Input: part model. Units: mm. Frame: model coordinates. A direction names the side the tool comes from. Coordinates: 2 decimals unless noted, no trailing zeros. Order: outer loops, then holes, each group sorted by start corner. A loop starts at its lowest first (then second) coordinate and runs counter-clockwise, first axis right, second up.
from build123d import *

# Parameters (mm, degrees)
SKETCH1_R               = 1.375
BOSS_EXTRUDE1_DEPTH     = 6.25
CUT_EXTRUDE1_DEPTH      = 15.811313244
CUT_EXTRUDE1_DEPTH_BACK = 15.811313244
SKETCH2_W               = 8
SKETCH2_H               = 6.5
BOSS_EXTRUDE2_START     = -10
BOSS_EXTRUDE2_OUTLINE_W = 11.434309127
BOSS_EXTRUDE2_OUTLINE_H = 8.5
BOSS_EXTRUDE2_DEPTH     = 20
FILLET4_R               = 1.5
FILLET5_R               = 1.5
FILLET6_R               = 3
CUT_EXTRUDE2_DEPTH      = 0.1


# Read off the part's stored shape, not the designer's step: Boss-Extrude2
with BuildPart() as part:
    # Sketch1 → Boss-Extrude1 (new, symmetric)
    with BuildSketch(Plane.XY):
        with BuildLine():
            Line((-10, 5.5), (-10, -3))
            Line((-10, -3), (8, -3))
            ThreePointArc((8, -3), (12.25, 1.25), (8, 5.5))
            Line((8, 5.5), (-10, 5.5))
        make_face()
        with Locations((8, 1.25)):
            Circle(SKETCH1_R, mode=Mode.SUBTRACT)
    extrude(amount=BOSS_EXTRUDE1_DEPTH, both=True)

    # Sketch2 → Cut-Extrude1 (cut, two sides: drawn at the far end of the back side and taken through both)
    with BuildSketch(Plane(origin=(0, 0, 0), x_dir=(1, 0, 0), z_dir=(0, 1, 0)).offset(-CUT_EXTRUDE1_DEPTH_BACK)):
        with Locations((8.25, 1)):
            Rectangle(SKETCH2_W, SKETCH2_H)
    extrude(amount=CUT_EXTRUDE1_DEPTH + CUT_EXTRUDE1_DEPTH_BACK, mode=Mode.SUBTRACT)

    # Boss-Extrude2 outline → Boss-Extrude2 (add)
    with BuildSketch(Plane.XY.offset(BOSS_EXTRUDE2_START)):
        with Locations((-4.282845436, 1.25)):
            Rectangle(BOSS_EXTRUDE2_OUTLINE_W, BOSS_EXTRUDE2_OUTLINE_H)
    extrude(amount=BOSS_EXTRUDE2_DEPTH)

    # Sketch1<5> → Cut-Revolve2 (revolve, cut)
    with BuildSketch(Plane.XY):
        with BuildLine():
            Line((-9.391951793, 2.5), (-10, 2.5))
            Line((-10, 2.5), (-10, 0))
            Line((-10, 0), (-7.720367157, 0))
            ThreePointArc((-7.720367157, 0), (-7.220367157, 0.5), (-6.720367157, 0))
            Line((-6.720367157, 0), (-2.720367157, 0))
            ThreePointArc((-2.720367157, 0), (-2.220367157, 0.5), (-1.720367157, 0))
            Line((-1.720367157, 0), (0, 0))
            Line((0, 0), (0, 2.5))
            Line((0, 2.5), (-3.391951793, 2.5))
            ThreePointArc((-3.391951793, 2.5), (-3.891951793, 2), (-4.391951793, 2.5))
            Line((-4.391951793, 2.5), (-8.391951793, 2.5))
            ThreePointArc((-8.391951793, 2.5), (-8.891951793, 2), (-9.391951793, 2.5))
        make_face()
    revolve(axis=Axis((-50, 0, 0), (0, 1, 0)), mode=Mode.SUBTRACT)

    # Fillet4
    fillet4_edges = [part.edges().sort_by_distance(p)[0] for p in [
        (4.25, 1.25, 2.25),
        (4.25, 1.25, -4.25),
    ]]
    fillet(fillet4_edges, radius=FILLET4_R)

    # Fillet5
    fillet5_edges = [part.edges().sort_by_distance(p)[0] for p in [
        (1.434309127, 1.25, -6.25),
        (1.434309127, 1.25, 6.25),
        (-1.010205144, 1.25, 10),
        (-1.010205144, 1.25, -10),
    ]]
    fillet(fillet5_edges, radius=FILLET5_R)

    # Fillet6
    fillet6_edges = [part.edges().sort_by_distance(p)[0] for p in [
        (-10, -1.5, -10),
        (-10, 3.757683564, -10),
        (-10, -1.5, 10),
        (-10, 3.757683564, 10),
    ]]
    fillet(fillet6_edges, radius=FILLET6_R)

    # Sketch5 → Cut-Extrude2 (cut)
    with BuildSketch(Plane(origin=(0, 5.5, 0), x_dir=(1, 0, 0), z_dir=(0, 1, 0))):
        with BuildLine():
            Line((-10, 0.5), (-5, 0.5))
            ThreePointArc((-5, 0.5), (-4.5, 0), (-5, -0.5))
            Line((-5, -0.5), (-10, -0.5))
            Line((-10, -0.5), (-10, 0.5))
        make_face()
    extrude(amount=-CUT_EXTRUDE2_DEPTH, mode=Mode.SUBTRACT)


solid = part.part
Item 1: Pin query (flat end, axial travel): pin 1 Ø2.5 at (y, z) = (1.5, 8.5) entering from +X; pin 2 Ø3 at (y, z) = (0.5, -1) entering from +X; pin 3 Ø2 at (x, y) = (7.5, 0) entering from -Z. Return the tip coordinate at first contact, or that it passes through.
Response values:
pin 1: stops at x = 1.52
pin 2: stops at x = 4.25
pin 3: stops at z = -6.25
Item 2: Cut plane A-A on y = 1.25. Return loops of the section in (x, z) (3 decimals), then the cut area to 3 significant figures.
Response values:
outline: (-0.686, -8.252) arc R1.5 ccw to (0.794, -10) - (1.434, -10) - (1.434, -7.75) arc R1.5 cw to (2.934, -6.25) - (6.625, -6.25) - (6.625, -4.25) - (5.75, -4.25) arc R1.5 cw to (4.25, -2.75) - (4.25, 0.75) arc R1.5 cw to (5.75, 2.25) - (6.625, 2.25) - (6.625, 6.25) - (2.934, 6.25) arc R1.5 cw to (1.434, 7.75) - (1.434, 10) - (0.794, 10) arc R1.5 ccw to (-0.686, 8.252) arc R50 cw to start; (9.375, -6.25) - (12.25, -6.25) - (12.25, -4.25) - (9.375, -4.25) - close; (9.375, 2.25) - (12.25, 2.25) - (12.25, 6.25) - (9.375, 6.25) - close
area: 103 mm2
Item 3: Draft query along Y for faces 6 (the face through (0, 1, 0)), 7 (the face through (12.25, 1.16, -5.24)), 8 (the face through (-10, -2, 0)). Return one class per face: pulls with the +Y half, pulls with the -Y half, needs draft (parallel to the pull), parting line crosses it, or undercut.
Response values:
face 6: undercut
face 7: parting line crosses it
face 8: needs draft
Item 4: Cut plane D-D on x = -0.25. Return loops of the section in (y, z).
Response values:
outline: (-3, -10) - (0, -10) - (0, -9.58) - (2.5, -9.58) - (2.5, -10) - (5.5, -10) - (5.5, 10) - (2.5, 10) - (2.5, 9.58) - (0, 9.58) - (0, 10) - (-3, 10) - close; hole (0, -4.99) - (2.5, -4.99) - (2.5, 4.99) - (0, 4.99) - close
Item 5: Access query for faces 1 (the face through (6, 1, -6.25)), 2 (the face through (-9, 0, 0)), 3 (the face through (10, 1, -4.25)), 4 (the face through (6, 1, 6.25)), 5 (the face through (-7, 5.4, 0)). Directions: +Z, -Z, +X, -X, +Y, -Y. A direction counts if a zero-diameter tool reaches every point of the face in a straight line with its end or side. Return the directions, or none.
Response values:
face 1: -Z, +X, +Y, -Y
face 2: -X
face 3: +X, +Y, -Y
face 4: +Z, +X, +Y, -Y
face 5: -X, +Y
Item 6: Cut plane B-B on z = 0. Return loops of the section in (x, y), then the cut area to 3 significant figures.
Response values:
outline: (-10, -3) - (4.25, -3) - (4.25, 5.5) - (-4.5, 5.5) - (-4.5, 5.4) - (-10, 5.4) - (-10, 2.5) - (-9.39, 2.5) arc R0.5 ccw to (-8.39, 2.5) - (-4.39, 2.5) arc R0.5 ccw to (-3.39, 2.5) - (0, 2.5) - (0, 0) - (-1.72, 0) arc R0.5 ccw to (-2.72, 0) - (-6.72, 0) arc R0.5 ccw to (-7.72, 0) - (-10, 0) - close
area: 97.1 mm2
Item 7: Cut plane C-C on x = 4.5. Return loops of the section in (y, z).
Response values:
outline: (-3, -6.25) - (5.5, -6.25) - (5.5, -3.58) - (-3, -3.58) - close; (-3, 1.58) - (5.5, 1.58) - (5.5, 6.25) - (-3, 6.25) - close
Item 8: Ray query, probe 1 along Y at (x, z) = (8, 3.55) (3 decimals); probe 2 along Y at (x, z) = (-8, -3); probe 3 along Z at (x, y) = (8.5, 4.5). Return the intervals inside material, ascending.
Response values:
probe 1: y = -3 to -0.125, 2.625 to 5.5
probe 2: y = -3 to 0, 2.5 to 5.5
probe 3: z = -6.25 to -4.25, 2.25 to 6.25
